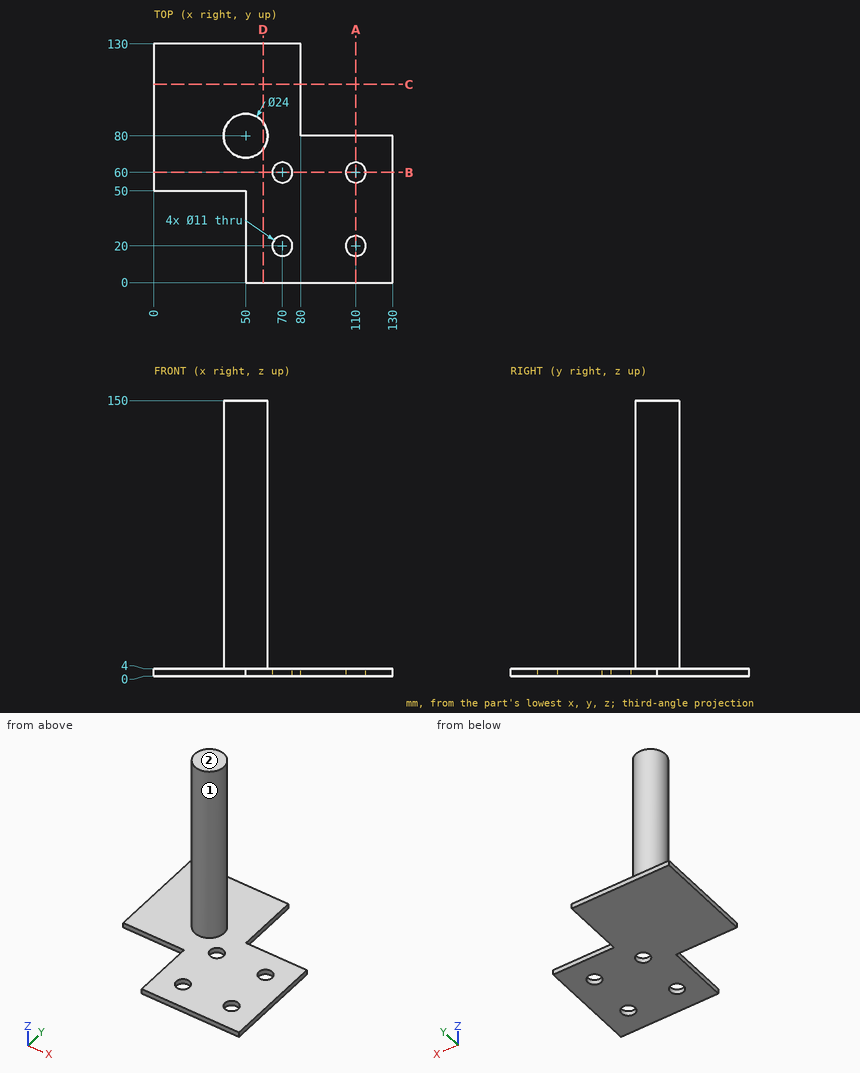
Source: three-view drawing plus pictorial views. Frame: mm from the lowest corner of the part. A direction names the side the tool comes from. Round coordinates to 2 decimals unless told otherwise and drop trailing zeros. Loops run counter-clockwise (first coordinate to the right, second up) from the corner with the lowest first, then second, coordinate; pieces in that order, holes last.
Q1. Pin query (flat end, axial travel): P1, Ø2, axis at y = 111, z = 2, coming from the +X side; P2, Ø4.5, axis at x = 95.5, z = 2, coming from the +Y side; P3, Ø2, axis at x = 39.5, z = 62, coming from the +Y side; P4, Ø6.5, axis at x = 70, y = 20, coming from the -Z side. Return the tip coordinate at first contact, or that it passes through.
Q2. Section A-A on x = 110. Return loops of the section in (y, z), plus the area to 3 significant figures.
Q3. Section D-D on x = 59.5. Return loops of the section in (y, z).
Q4. Access query for the marked faces 1 and 2. Directions: +Z, -Z, +X, -X, +Y, -Y. A direction counts if a zero-diameter tool reaches every point of the face in a straight line with its end or side. Return the directions, or none.
Q5. Section B-B on y = 60. Return loops of the section in (x, z), plus the area to 3 significant figures.
Q6. Section C-C on y = 108. Return loops of the section in (x, z).
Q7. Material intervals for L1, parallel to Y at x = 110, z = 1.7; L2, parallel to Y at x = 70, z = 2; L3, parallel to Z at x = 82, y = 35, sorted ascending.
Evaluation:
1. P1: stops at x = 80
1. P2: stops at y = 80
1. P3: stops at y = 87.33
1. P4: passes through
2. outline: (0, 0) - (14.5, 0) - (14.5, 4) - (0, 4) - close; (25.5, 0) - (54.5, 0) - (54.5, 4) - (25.5, 4) - close; (65.5, 0) - (80, 0) - (80, 4) - (65.5, 4) - close
2. area: 232 mm2
3. outline: (0, 0) - (130, 0) - (130, 4) - (87.33, 4) - (87.33, 150) - (72.67, 150) - (72.67, 4) - (0, 4) - close
4. face 1: +Z
4. face 2: +Z, +X, -X, +Y, -Y
5. outline: (0, 0) - (64.5, 0) - (64.5, 4) - (0, 4) - close; (75.5, 0) - (104.5, 0) - (104.5, 4) - (75.5, 4) - close; (115.5, 0) - (130, 0) - (130, 4) - (115.5, 4) - close
5. area: 432 mm2
6. outline: (0, 0) - (80, 0) - (80, 4) - (0, 4) - close
7. L1: y = 0 to 14.5, 25.5 to 54.5, 65.5 to 80
7. L2: y = 0 to 14.5, 25.5 to 54.5, 65.5 to 130
7. L3: z = 0 to 4
